Part model, mm, in its own coordinate system. Face numbers are marked on the shaded views. Round coordinates to 2 decimals unless told otherwise and drop trailing zeros. Write each loop counter-clockwise with the first axis right and the second up, starting at its lowest first coordinate (ties: lowest second). Pieces come first, ordered by that corner, then holes.
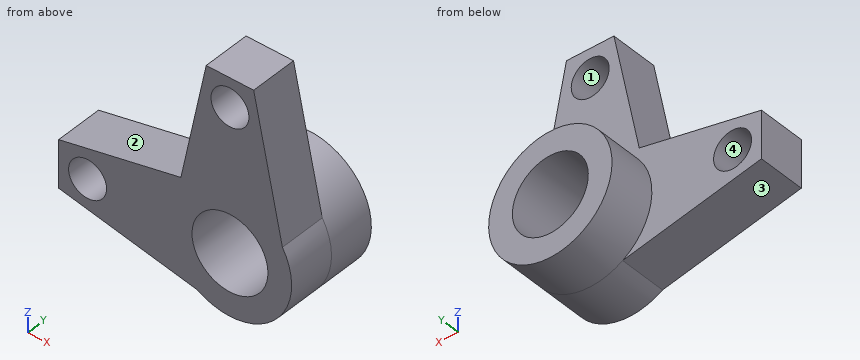
```python
from build123d import *

# Parameters (mm, degrees)
SKETCH1_R           = 2
SKETCH1_R_2         = 4
BOSS_EXTRUDE1_DEPTH = 5
SKETCH1_3_R         = 6.5
SKETCH1_3_R_2       = 4
BOSS_EXTRUDE2_DEPTH = 10


with BuildPart() as part:
    # Sketch1 → Boss-Extrude1 (new body)
    with BuildSketch(Plane(origin=(0, 0, 0), x_dir=(1, 0, 0), z_dir=(0, 1, 0))):
        with BuildLine():
            Line((-3.418800465, 5.528273092), (-18.046143069, 2.5))
            Line((-18.046143069, 2.5), (-18.046143069, -2.5))
            Line((-18.046143069, -2.5), (-5.166458511, -5.166458511))
            Line((-5.166458511, -5.166458511), (-2.5, -18.046143069))
            Line((-2.5, -18.046143069), (2.5, -18.046143069))
            Line((2.5, -18.046143069), (5.528273092, -3.418800465))
            ThreePointArc((5.528273092, -3.418800465), (4.596194078, 4.596194078), (-3.418800465, 5.528273092))
        make_face()
        with Locations(Location((-15, 0, 0), (0, 0, 270))):
            Circle(SKETCH1_R, mode=Mode.SUBTRACT)
        with Locations(Location((0, 0, 0), (0, 0, 270))):
            Circle(SKETCH1_R_2, mode=Mode.SUBTRACT)
        with Locations(Location((0, -15, 0), (0, 0, 270))):
            Circle(SKETCH1_R, mode=Mode.SUBTRACT)
    extrude(amount=BOSS_EXTRUDE1_DEPTH)

    # Sketch1<3> → Boss-Extrude2 (add)
    with BuildSketch(Plane(origin=(0, 0, 0), x_dir=(1, 0, 0), z_dir=(0, 1, 0))):
        with Locations(Location((0, 0, 0), (0, 0, 121.733519153))):
            Circle(SKETCH1_3_R)
        with Locations(Location((0, 0, 0), (0, 0, 270))):
            Circle(SKETCH1_3_R_2, mode=Mode.SUBTRACT)
    extrude(amount=BOSS_EXTRUDE2_DEPTH)


solid = part.part
```
Q1. Cut at C-C on x = 0. Write the cut outline in (y, z), plus the area to 3 significant figures.
Values follow:
outline: (0, -6.5) - (10, -6.5) - (10, -4) - (0, -4) - close; (0, 4) - (10, 4) - (10, 6.5) - (5, 6.5) - (5, 13) - (0, 13) - close; (0, 17) - (5, 17) - (5, 18.05) - (0, 18.05) - close
area: 87.7 mm2
Q2. Cut at B-B on y = 3. Write the cut outline in (x, z).
Values follow:
outline: (-18.05, -2.5) - (-3.42, -5.53) arc R6.5 ccw to (5.53, 3.42) - (2.5, 18.05) - (-2.5, 18.05) - (-5.17, 5.17) - (-18.05, 2.5) - close; hole circle Ø4 at (-15, 0); hole circle Ø8 at (0, 0); hole circle Ø4 at (0, 15)
Q3. Wall check: L1, parallel to X at y = 4.5, z = 0; L2, parallel to X at y = 2, z = 1.5; L3, parallel to Z at x = 0.75, y = 4.5. Give the ranges that are in metal, low to high.
Values follow:
L1: x = -18.05 to -17, -13 to -4, 4 to 6.5
L2: x = -18.05 to -16.32, -13.68 to -3.71, 3.71 to 6.32
L3: z = -6.46 to -3.93, 3.93 to 13.15, 16.85 to 18.05
Q4. Cut at D-D on z = 15. Write the cut outline in (x, y), plus the area to 3 significant figures.
Values follow:
outline: (-3.13, 0) - (-2, 0) - (-2, 5) - (-3.13, 5) - close; (2, 0) - (3.13, 0) - (3.13, 5) - (2, 5) - close
area: 11.3 mm2
Q5. Drop a flat-ended pin along its axis: pin 1 (4 mm diameter, centred on y = 6, z = 10, fed in from +X). Give the stop position or say it passes through.
Values follow:
pin 1: stops at x = 4.52
Q6. Cut at A-A on z = 0. Write the cut outline in (x, y), plus the area to 3 significant figures.
Values follow:
outline: (-18.05, 0) - (-17, 0) - (-17, 5) - (-18.05, 5) - close; (-13, 0) - (-4, 0) - (-4, 10) - (-6.5, 10) - (-6.5, 5) - (-13, 5) - close; (4, 0) - (6.5, 0) - (6.5, 10) - (4, 10) - close
area: 87.7 mm2
Q7. Mould opens along Z. For the marked faces 1, 2, 3 and 4 say: +Z half, -Z half, draft (parallel to the pull), parting line (faces both ways), or undercut.
Values follow:
face 1: undercut
face 2: +Z half
face 3: -Z half
face 4: undercut
